Autodesk Fusion 360 part; units mm, degrees
sketch "Sketch1" plane through (0, 0, 0) normal (0, 1, 0) x (1, 0, 0)
  line L0 (76.2, 38.1) -> (-76.2, 38.1)
  line L1 (-76.2, 38.1) -> (-76.2, -38.1)
  line L2 (-76.2, -38.1) -> (76.2, -38.1)
  line L3 (76.2, -38.1) -> (76.2, 38.1)
  line L4 (76.2, 38.1) -> (-76.2, -38.1) construction
  line L5 (-76.2, 38.1) -> (76.2, -38.1) construction
  dimension "d1" = 76.2
  dimension "d2" = 152.4
extrude "Extrude1" add sketch "Sketch1" along normal blind 25.4
ref_plane "WorkPlane1" through (0, 38.1, 0) normal (0, 1, 0) x (0, 0, 1)
sketch "Sketch3" plane through (0, 38.1, 0) normal (0, 1, 0) x (1, 0, 0)
  circle A0 centre (0, 0) radius 19.05
  dimension "d6" = 38.1
sketch "Sketch4" plane through (0, 25.4, 0) normal (0, 1, 0) x (-1, 0, 0)
  line L0 (-76.2, 38.1) -> (-76.2, -38.1)
  line L1 (-76.2, -38.1) -> (76.2, -38.1)
  line L2 (76.2, -38.1) -> (76.2, 38.1)
  line L3 (76.2, 38.1) -> (-76.2, 38.1)
  circle A0 centre (0, 0) radius 34.925
  dimension "d7" = 69.85
loft "Loft1" add profiles "Sketch4", "Sketch3" section 1 contours A0 section 2
fillet "Fillet1" radius 3.175 2 edges at (-17.7608, 38.1, -6.8888) (32.5615, 25.4, 12.6294)
sketch "Sketch5" plane through (0, 25.4, 0) normal (0, 1, 0) x (-1, 0, 0)
  line L0 (-76.2, 38.1) -> (-76.2, -38.1)
  line L1 (-76.2, -38.1) -> (76.2, -38.1)
  line L2 (76.2, -38.1) -> (76.2, 38.1)
  line L3 (76.2, 38.1) -> (-76.2, 38.1)
  circle A0 centre (0, 0) radius 36.0387
  line L4 (76.2, 0) -> (-76.2, 0) construction
  line L5 (-76.2, -21.9448) -> (-50.8, -12.7)
  line L6 (-50.8, -12.7) -> (-50.8, 12.7)
  line L7 (-50.8, 12.7) -> (-76.2, 21.9448)
  line L8 (0, 0) -> (0, -47.7527) construction
  line L9 (50.8, 12.7) -> (76.2, 21.9448)
  line L10 (50.8, -12.7) -> (50.8, 12.7)
  line L11 (76.2, -21.9448) -> (50.8, -12.7)
  dimension "d10" = 25.4
  dimension "d11" = 25.4
  dimension "d12" = 70
extrude "Extrude2" cut sketch "Sketch5" against normal blind 6.35 contours L0 L5 L6 L7 | L2 L9 L10 L11
fillet "Fillet2" radius 7.62 8 edges at (76.2, 22.225, -21.9448) (76.2, 22.225, 21.9448) (50.8, 22.225, -12.7) (50.8, 22.225, 12.7) (-50.8, 22.225, 12.7) (-50.8, 22.225, -12.7) (-76.2, 22.225, -21.9448) (-76.2, 22.225, 21.9448)
sketch "Sketch6" plane through (0, 38.1, 0) normal (0, 1, 0) x (-1, 0, 0)
  circle A0 centre (0, 0) radius 17.9363
  circle A1 centre (0, -7.62) radius 7.62
  circle A2 centre (6.5991, 3.81) radius 7.62
  circle A3 centre (-6.5991, 3.81) radius 7.62
  dimension "d16" = 15.24
  dimension "d17" = 7.62
  dimension "d19" = 360
extrude "Extrude3" cut sketch "Sketch6" against normal blind 6.35 contours A1 A2 A3 | A1 A2 | A1 A2 A3 | A1 A2 A3 | A1 A3 | A2 A3
fillet "Fillet3" radius 2.54 3 edges at (-6.5991, 34.925, -3.81) (6.5991, 34.925, -3.81) (0, 34.925, 7.62)
chamfer "Chamfer2" distance 0.635 angle 45 4 edges at (76.2, 12.7, 38.1) (-76.2, 12.7, 38.1) (-76.2, 12.7, -38.1) (76.2, 12.7, -38.1)
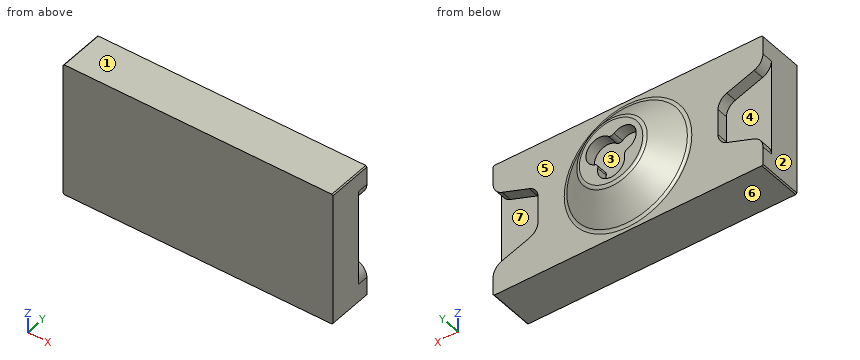
Input: part model. Units: mm. Frame: model coordinates. Face numbers are marked on the shaded views. A direction names the side the tool comes from. Give positions to 0.01 mm unless a question says otherwise; leave off trailing zeros. Loops run counter-clockwise (first coordinate to the right, second up) from the corner with the lowest first, then second, coordinate; pieces in that order, holes last.
1) Contact query for flat-ended pins moving along their axis: pin 1 (5 mm diameter, centred on y = 23.5, z = 1.5, fed in from +X); pin 2 (12 mm diameter, centred on x = -6.6, z = 3.81, fed in from +Y); pin 3 (3 mm diameter, centred on y = 29.5, z = -13.5, fed in from +X). Output: stop coordinate, or through.
A:
pin 1: stops at x = 50.8
pin 2: stops at y = 31.75
pin 3: stops at x = 28.77
2) Section query A-A on x = -64. Return the cut outline in (y, z).
A:
outline: (0, -38.1) - (25.4, -38.1) - (25.4, -17.5) - (19.05, -17.5) - (19.05, 17.5) - (25.4, 17.5) - (25.4, 38.1) - (0, 38.1) - close
3) Line query: L1, parallel to Y at x = -41, z = 17.5; L2, parallel to Y at x = 10, z = 3; L3, parallel to Z at x = 0, y = 33.5. Output: solid intervals per line, ascending.
A:
L1: y = 0 to 25.4
L2: y = 0 to 31.75
L3: z = -24.8 to -15.24, 9 to 24.8
4) Reachability of the marked faces 4, 5, 6 and 7 from +Z, -Z, +X, -X, +Y, -Y: full face, straight path, thin tool, end or side. Return the list, or none.
A:
face 4: -X, +Y
face 5: +Y
face 6: -Z, +X, -X, +Y, -Y
face 7: +X, +Y
5) Section query C-C on x = -44.5. Return the cut outline in (y, z).
A:
outline: (0, -38.1) - (25.4, -38.1) - (25.4, 38.1) - (0, 38.1) - close
6) Mould query, pull axis X, two halves, no side actions, for the marked faces 1, 2 and 3. Classes: released by +X, released by -X, zero draft, split by the parting line, or undercut.
A:
face 1: zero draft
face 2: released by -X
face 3: undercut
7) Section query B-B on y = 28. Return the cut outline in (x, z) (3 decimals).
A:
outline: circle Ø63.35 at (0, 0)
